The listing builds one solid part. Answer for the finished solid, in the listing's coordinates (mm). Face numbers are marked on the shaded views. A direction names the side the tool comes from. Give positions to 0.01 mm unless a question says otherwise; leave off trailing zeros. Order: outer loops, then holes, each group sorted by start corner. A loop starts at its lowest first (then second) coordinate and runs counter-clockwise, first axis right, second up. Notation, with made-up numbers: (65, 45.5) - (110, 45.5) arc R19 cw to (110, 61.5) - close; hole circle Ø11 at (-19.75, 85). An arc over 180 degrees is marked (long way). Answer as a JSON object with one key per item and string values. Group by question number.
Q1. A cutting plane is placed at B-B, the plane y = 42. Give the vertices of the cut face in (x, z), and give its area (3 significant figures).
Q2. Consider line 1 (Z direction, x = 0, y = 30) (3 decimals); line 2 (Z direction, x = 0, y = 15.5); line 3 (X direction, y = -10, z = -7). Determine where each line is inside the solid, lowest interval first.
Q3. A cutting plane is placed at A-A, the plane x = 0. Give the vertices of the cut face in (y, z) (3 decimals).
Q4. For the marked faces 1 and 2, determine the directions among +Z, -Z, +X, -X, +Y, -Y from which every point of the face is accessible in a straight line to the end or side of a thin tool.
Q5. Given pin 1 (5 mm diameter, centred on y = 36.5, z = 5, fed in from -X); pin 2 (3 mm diameter, centred on x = 25, y = 30.5, fed in from -Z); pin 3 (12 mm diameter, centred on x = -14.5, z = 2.5, fed in from +Y), each flat-ended and moving along its own axis, determine where each tip first touches the part or whether it passes through.
Q6. A cutting plane is placed at C-C, the plane z = 8.75. Give the vertices of the cut face in (x, y).
Q7. A cutting plane is placed at D-D, the plane z = 15.5. Give the vertices of the cut face in (x, y).
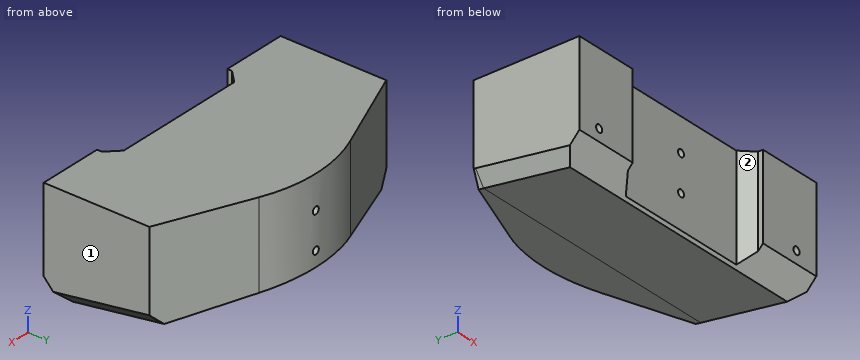
from build123d import *

# Parameters (mm, degrees)
CROQUIS1_W              = 120
CROQUIS1_H              = 45
CROQUIS1_R              = 1.55
SALIENTE_EXTRUIR1_DEPTH = 30
CROQUIS2_W              = 120
CROQUIS2_H              = 45
SALIENTE_EXTRUIR2_DEPTH = 44
SALIENTE_EXTRUIR5_DEPTH = 45
CROQUIS6_R              = 1.55
CORTAR_EXTRUIR2_DEPTH   = 6
CORTAR_EXTRUIR3_DEPTH   = 132.932747906
CHAFL_N1_SIZE           = 5
CROQUIS9_W              = 66
CROQUIS9_H              = 7
CORTAR_EXTRUIR4_DEPTH   = 91.138781721
CHAFL_N2_SIZE           = 5
CORTAR_EXTRUIR6_DEPTH   = 132.932747906
CROQUIS11_R             = 1.5
CORTAR_EXTRUIR7_DEPTH   = 86.762753955


with BuildPart() as part:
    # Croquis1 → Saliente-Extruir1 (new body)
    with BuildSketch(Plane(origin=(0, 0, 0), x_dir=(1, 0, 0), z_dir=(0, 1, 0))):
        Rectangle(CROQUIS1_W, CROQUIS1_H)
        with Locations(Location((-50, -7.5, 0), (0, 0, 270))):
            Circle(CROQUIS1_R, mode=Mode.SUBTRACT)
        with Locations(Location((50, -7.5, 0), (0, 0, 270))):
            Circle(CROQUIS1_R, mode=Mode.SUBTRACT)
    extrude(amount=SALIENTE_EXTRUIR1_DEPTH)

    # Croquis2 → Saliente-Extruir2 (add)
    with BuildSketch(Plane(origin=(0, 30, 0), x_dir=(1, 0, 0), z_dir=(0, 1, 0))):
        Rectangle(CROQUIS2_W, CROQUIS2_H)
    extrude(amount=-SALIENTE_EXTRUIR2_DEPTH)

    # Croquis5 → Saliente-Extruir5 (add, through all)
    with BuildSketch(Plane.XY.offset(22.5)):
        with BuildLine():
            Line((-60, 30), (-23.076922962, 45.384615109))
            ThreePointArc((-23.076922962, 45.384615109), (0, 49.999999701), (23.076922962, 45.384615109))
            Line((23.076922962, 45.384615109), (60, 30))
            Line((60, 30), (-60, 30))
        make_face()
    extrude(amount=-SALIENTE_EXTRUIR5_DEPTH)

    # Croquis6 → Cortar-Extruir2 (cut)
    with BuildSketch(Plane.XZ.offset(14)):
        with Locations(Location((-50, -7.5, 0), (0, 0, 270))):
            Circle(CROQUIS6_R)
        with Locations(Location((50, -7.5, 0), (0, 0, 270))):
            Circle(CROQUIS6_R)
    extrude(amount=-CORTAR_EXTRUIR2_DEPTH, mode=Mode.SUBTRACT)

    # Croquis8 → Cortar-Extruir3 (cut, through all)
    with BuildSketch(Plane.ZY.offset(60)):
        Polygon((-22.5, 30), (-15.624999968, 30), (-12.5, 49.999999701), (-22.5, 49.999999701), align=None)
        Polygon((-22.5, 30), (-22.5, -14), (-15.624999968, 30), align=None)
    extrude(amount=-CORTAR_EXTRUIR3_DEPTH, mode=Mode.SUBTRACT)

    # Chaflán1
    chafl_n1_edges = [part.edges().sort_by_distance(p)[0] for p in [
        (60, 8, -19.062499984),
        (-60, 8, -19.062499984),
    ]]
    chamfer(chafl_n1_edges, length=CHAFL_N1_SIZE)

    # Croquis9 → Cortar-Extruir4 (cut, through all)
    with BuildSketch(Plane.XY.offset(22.5)):
        with Locations((0, -10.5)):
            Rectangle(CROQUIS9_W, CROQUIS9_H)
    extrude(amount=-CORTAR_EXTRUIR4_DEPTH, mode=Mode.SUBTRACT)

    # Chaflán2
    chafl_n2_edges = [part.edges().sort_by_distance(p)[0] for p in [
        (-33, -7, 0.546875003),
        (33, -7, 0.546875003),
    ]]
    chamfer(chafl_n2_edges, length=CHAFL_N2_SIZE)

    # Croquis10 → Cortar-Extruir6 (cut, through all)
    with BuildSketch(Plane.ZY.offset(60)):
        Polygon((-21.249999994, -6), (-12.5, -14), (-22.5, -14), align=None)
    extrude(amount=-CORTAR_EXTRUIR6_DEPTH, mode=Mode.SUBTRACT)

    # Croquis11 → Cortar-Extruir7 (cut, through all)
    with BuildSketch(Plane.XZ.offset(7)):
        with Locations(Location((0, -6.249999994, 0), (0, 0, 270))):
            Circle(CROQUIS11_R)
        with Locations(Location((0, 8.750000006, 0), (0, 0, 270))):
            Circle(CROQUIS11_R)
    extrude(amount=-CORTAR_EXTRUIR7_DEPTH, mode=Mode.SUBTRACT)


solid = part.part
Reply:
{
 "1": {"outline": "(-31.2, -13.75) - (31.2, -13.75) - (31.2, 22.5) - (-31.2, 22.5) - close; hole circle Ø3 at (0, -6.25); hole circle Ø3 at (0, 8.75)", "area": "2,250 mm^2"},
 "2": {"line 1": "z = -15.625 to -7.75, -4.75 to 7.25, 10.25 to 22.5", "line 2": "z = -17.89 to -7.75, -4.75 to 7.25, 10.25 to 22.5", "line 3": "x = -60 to -51.47, -48.53 to -31, 31 to 48.53, 51.47 to 60"},
 "3": {"outline": "(-7, -20.156) - (-6, -21.25) - (50, -12.5) - (50, -7.75) - (-7, -7.75) - close; (-7, -4.75) - (50, -4.75) - (50, 7.25) - (-7, 7.25) - close; (-7, 10.25) - (50, 10.25) - (50, 22.5) - (-7, 22.5) - close"},
 "4": {"face 1": "+Z, -Z, +X, +Y, -Y", "face 2": "+Z, -Z, -Y"},
 "5": {"pin 1": "stops at x = -50.4", "pin 2": "stops at z = -15.78", "pin 3": "stops at y = 49.39"},
 "6": {"outline": "(-60, -14) - (-33, -14) - (-33, -12) - (-28, -7) - (-1.5, -7) - (-1.5, 49.98) arc R60 ccw to (-23.08, 45.38) - (-60, 30) - close; (1.5, -7) - (28, -7) - (33, -12) - (33, -14) - (60, -14) - (60, 30) - (23.08, 45.38) arc R60 ccw to (1.5, 49.98) - close"},
 "7": {"outline": "(-60, -14) - (-33, -14) - (-33, -12) - (-28, -7) - (28, -7) - (33, -12) - (33, -14) - (60, -14) - (60, 30) - (23.08, 45.38) arc R60 ccw to (-23.08, 45.38) - (-60, 30) - close"}
}
